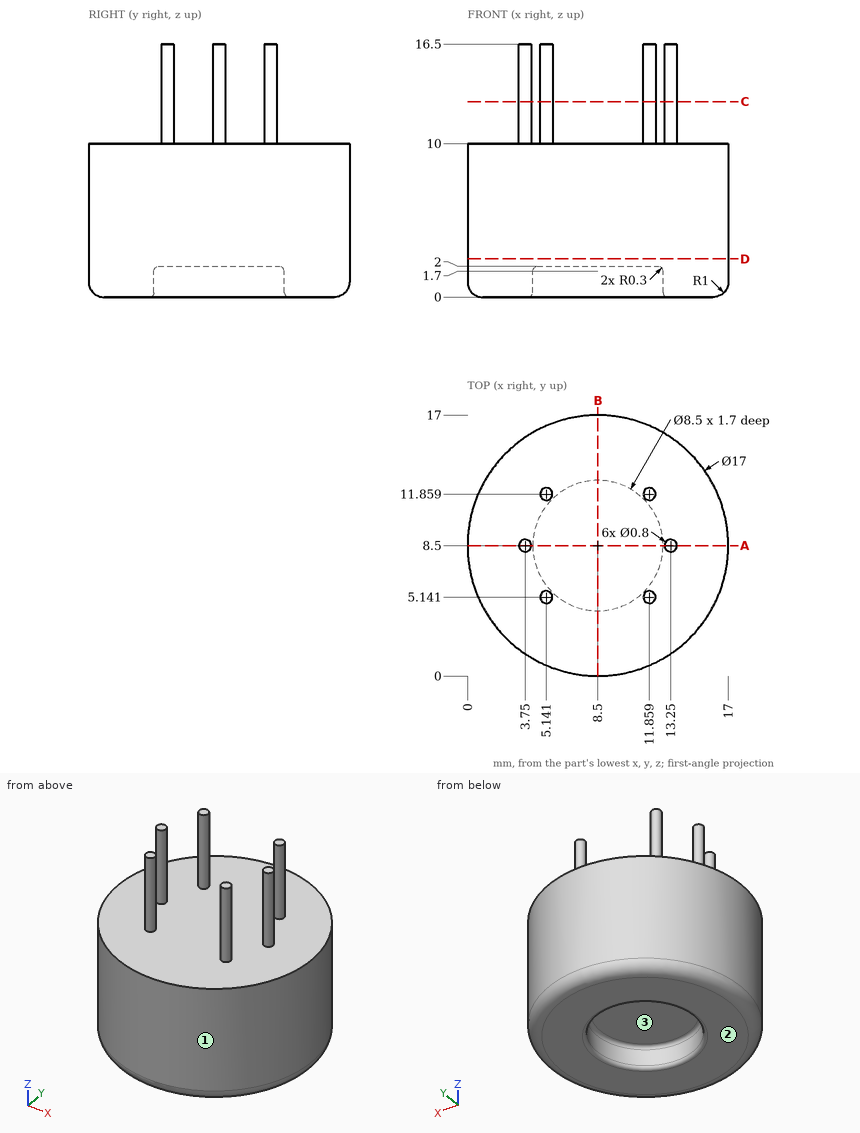
Drawing for the job (mm, zero at the part's lowest x, y, z). Round coordinates to 2 decimals unless told otherwise and drop trailing zeros. Write each loop counter-clockwise with the first axis right and the second up, starting at its lowest first coordinate (ties: lowest second). Pieces come first, ordered by that corner, then holes.
Item 1: Band-saw the part on B-B on x = 8.5. Write the cut outline in (y, z).
Filled in:
outline: (0, 1) arc R1 ccw to (1, 0) - (3.95, 0) arc R0.3 ccw to (4.25, 0.3) - (4.25, 1.7) arc R0.3 cw to (4.55, 2) - (12.45, 2) arc R0.3 cw to (12.75, 1.7) - (12.75, 0.3) arc R0.3 ccw to (13.05, 0) - (16, 0) arc R1 ccw to (17, 1) - (17, 10) - (0, 10) - close
Item 2: Mould opens along X. For the marked faces 1, 2 and 3 say: released by +X, released by -X, zero draft, split by the parting line, or undercut.
Filled in:
face 1: split by the parting line
face 2: zero draft
face 3: undercut
Item 3: Drop flat-ended pins along their axis: pin 1 Ø1.5 at (x, z) = (5.5, 2) entering from -Y; pin 2 Ø3 at (x, y) = (5.5, 13) entering from +Z; pin 3 Ø4 at (x, y) = (10, 9.5) entering from -Z; pin 4 Ø3 at (x, z) = (3.5, 8.5) entering from +Y. Give the stop position or say it passes through.
Filled in:
pin 1: stops at y = 0.3
pin 2: stops at z = 16.5
pin 3: stops at z = 2
pin 4: stops at y = 16.25
Item 4: Band-saw the part on A-A on y = 8.5. Write the cut outline in (x, z), then the cut area to 3 significant figures.
Filled in:
outline: (0, 1) arc R1 ccw to (1, 0) - (3.95, 0) arc R0.3 ccw to (4.25, 0.3) - (4.25, 1.7) arc R0.3 cw to (4.55, 2) - (12.45, 2) arc R0.3 cw to (12.75, 1.7) - (12.75, 0.3) arc R0.3 ccw to (13.05, 0) - (16, 0) arc R1 ccw to (17, 1) - (17, 10) - (13.65, 10) - (13.65, 16.5) - (12.85, 16.5) - (12.85, 10) - (4.15, 10) - (4.15, 16.5) - (3.35, 16.5) - (3.35, 10) - (0, 10) - close
area: 163 mm2
Item 5: Band-saw the part on D-D on z = 2.5. Write the cut outline in (x, y).
Filled in:
outline: circle Ø17 at (8.5, 8.5)
Item 6: Drill centre lines: L1, parallel to Z at x = 7, y = 11.75; L2, parallel to Z at x = 5.75, y = 1.75; L3, parallel to Y at x = 8.5, z = 1.45. Where is each one in solid material? Low to high.
Filled in:
L1: z = 2 to 10
L2: z = 0 to 10
L3: y = 0 to 4.25, 12.75 to 17
Item 7: Band-saw the part on C-C on z = 12.75. Write the cut outline in (x, y).
Filled in:
outline: circle Ø0.8 at (3.75, 8.5); circle Ø0.8 at (5.14, 5.14); circle Ø0.8 at (5.14, 11.86); circle Ø0.8 at (11.86, 5.14); circle Ø0.8 at (11.86, 11.86); circle Ø0.8 at (13.25, 8.5)
